Input: part model. Units: mm. Frame: model coordinates. A direction names the side the tool comes from. Round coordinates to 2 decimals unless told otherwise and drop trailing zeros. Loops run counter-clockwise (first coordinate to the right, second up) from the corner with the lowest first, then second, coordinate; pieces in that order, holes last. Notation, with made-up numbers: (25.25, 49) - (54.25, 49) arc R13 ccw to (54.25, 67) - close; hole circle Ø6 at (-32.5, -32.75). An arc over 180 degrees is marked (long way). Use CSV: the item, a comma, the result in double quotes. Start each with the question number.
1. Cut plane A-A (y = 0). Return loops of the section in (x, z), and give its area (3 significant figures).
2. Material intervals for probe 1 along X at (y, z) = (0, 1.25); probe 2 along Y at (x, z) = (53, 2); probe 3 along Y at (x, z) = (3, 2.75), sorted ascending. Write a range as from..to.
3. Access query for faces 5 (the flat face through (17.783, -23.608, 0.07)), 6 (the cylindrical face through (-17.128, 0.295, 0.07)). Directions: +Z, -Z, +X, -X, +Y, -Y. A direction counts if a zero-diameter tool reaches every point of the face in a straight line with its end or side. Return the directions, or none.
4. Pin query (flat end, axial travel): P1, Ø10, axis at x = 0, y = -20, coming from the -Z side; P2, Ø1.5, axis at y = 12.5, z = -3.5, coming from the -X side; P3, Ø3, axis at x = 32.5, z = -0.5, coming from the +Y side; P4, Ø2, axis at x = 44, z = 0, coming from the +Y side. Return the tip coordinate at first contact, or that it passes through.
5. Cut plane C-C (z = 2.25). Return loops of the section in (x, y), and give its area (3 significant figures).
6. Pull-direction query (Y, two-part tool) for faces 1 (the cylindrical face through (-16.328, 0.281, 0.07)), 2 (the flat face through (17.516, -24.362, 0.07)), 3 (the flat face through (18.176, 24.595, 0.07)), 4 (the cylindrical face through (86.984, -0.909, 0.07)); classes: +Y half, -Y half, draft (parallel to the pull), parting line (faces both ways), or undercut.
7. Cut plane B-B (x = 17). Return loops of the section in (y, z), and give its area (3 significant figures).
Autodesk Inventor part; units mm, degrees
ref_plane "YZ Plane" through (0, 0, 0) normal (1, 0, 0) x (0, 1, 0)
ref_plane "XZ Plane" through (0, 0, 0) normal (0, 1, 0) x (-1, 0, 0)
ref_plane "XY Plane" through (0, 0, 0) normal (0, 0, 1) x (1, 0, 0)
sketch "スケッチ1" plane through (0, 0, 0) normal (0, 0, 1) x (1, 0, 0)
  arc A0 (-5.5703, 15.7556) -> (-5.5703, -15.7556) centre (0, 0) ccw
  arc A1 (41.5411, -32.4115) -> (41.5411, 32.4115) centre (53, 0) ccw
  line L0 (-5.5703, 15.7556) -> (41.5411, 32.4115)
  line L1 (-5.5703, -15.7556) -> (41.5411, -32.4115)
  line L2 (41.4015, 32.8065) -> (-5.7099, 16.1506)
  arc A2 (-5.7099, 16.1506) -> (-5.7099, -16.1506) centre (0, 0) ccw
  line L3 (-5.7099, -16.1506) -> (41.4015, -32.8065)
  arc A3 (41.4015, -32.8065) -> (41.4015, 32.8065) centre (53, 0) ccw
  line L4 (41.6681, 32.0523) -> (-5.4433, 15.3964)
  arc A4 (-5.4433, 15.3964) -> (-5.4433, -15.3964) centre (0, 0) ccw
  line L5 (-5.4433, -15.3964) -> (41.6681, -32.0523)
  arc A5 (41.6681, -32.0523) -> (41.6681, 32.0523) centre (53, 0) ccw
  dimension "d6" = 33.4225
  dimension "d7" = 68.7549
  dimension "d8" = 53
  dimension "d11" = 0.419
  dimension "d12" = 0.8
extrude "押し出し1" add sketch "スケッチ1" along normal mid plane 10 contours L0 A1 L1 A0 | A3 L3 A2 L2
properties part number "belt5" material "ゴム"
Established:
1,outline,"(-17.13, -5) - (-16.33, -5) - (-16.33, 5) - (-17.13, 5) - close; (87, -5) - (87.8, -5) - (87.8, 5) - (87, 5) - close"
1,area,"16.0 mm2"
2,probe 1,"x = -17.13..-16.33, 87..87.8"
2,probe 2,"y = -34.8..-34, 34..34.8"
2,probe 3,"y = -19.23..-18.38, 18.38..19.23"
3,face 5,"+Z, -Z"
3,face 6,"+Z, -Z, -X"
4,P1,"stops at z = -5"
4,P2,"stops at x = -12.47"
4,P3,"stops at y = 30.19"
4,P4,"stops at y = 33.86"
5,outline,"(-5.71, -16.15) - (41.4, -32.81) arc R34.8 ccw (long way) to (41.4, 32.81) - (-5.71, 16.15) arc R17.13 ccw to start; hole (-5.44, -15.4) - (41.67, -32.05) arc R34 ccw (long way) to (41.67, 32.05) - (-5.44, 15.4) arc R16.33 ccw to start"
5,area,"218 mm2"
6,face 1,"undercut"
6,face 2,"-Y half"
6,face 3,"+Y half"
6,face 4,"undercut"
7,outline,"(-24.18, -5) - (-23.33, -5) - (-23.33, 5) - (-24.18, 5) - close; (23.33, -5) - (24.18, -5) - (24.18, 5) - (23.33, 5) - close"
7,area,"17.0 mm2"
